Design review of the part built by this model. Coordinates are the model's own, in mm. A direction names the side the tool comes from. Give positions to 0.01 mm unless a question says otherwise; leave off trailing zeros. Order: outer loops, then holes, each group sorted by start corner. A loop starts at its lowest first (then second) coordinate and runs counter-clockwise, first axis right, second up. Notation, with made-up numbers: M 52.5,-28.5 L 95.5,-28.5 A29 cw 95.5,1.5 Z; hole C 24.25,-1.75 d4. An arc over 180 degrees is marked long. Answer as a JSON object with one key per item and string values.
from build123d import *

# Parameters (mm, degrees)
F0_R     = 25
F0_R_2   = 15
F1_DEPTH = 5
F2_DEPTH = 30
F3_R     = 10
F4_DEPTH = 15
F5_R     = 23
F6_DEPTH = 2


with BuildPart() as f1:
    # F0 (on Top) → F1 (new body)
    with BuildSketch(Plane.XY):
        Circle(F0_R)
        Circle(F0_R_2, mode=Mode.SUBTRACT)
    extrude(amount=F1_DEPTH)

    # F0 (on Top) → F2 (join)
    with BuildSketch(Plane.XY):
        Circle(F0_R_2)
    extrude(amount=F2_DEPTH)

    # F3 (on face) → F4 (cut)
    with BuildSketch(Plane.XY.offset(30)):
        Circle(F3_R)
    extrude(amount=-F4_DEPTH, mode=Mode.SUBTRACT)

    # F5 (on face) → F6 (cut)
    with BuildSketch(Plane.XY):
        Circle(F5_R)
    extrude(amount=F6_DEPTH, mode=Mode.SUBTRACT)


solid = f1.part
(1) We need section A-A (y = 0). Write out the cut boundary in (x, z), plus the area to 3 significant figures.
Checked values:
{"outline": "M -25,0 L -23,0 L -23,2 L 23,2 L 23,0 L 25,0 L 25,5 L 15,5 L 15,30 L 10,30 L 10,15 L -10,15 L -10,30 L -15,30 L -15,5 L -25,5 Z", "area": "608 mm^2"}
(2) We need section D-D (z = 9.75). Write out the cut boundary in (x, y).
Checked values:
{"outline": "C 0,0 d30"}
(3) Draft analysis for pull direction X (two halves, no side actions). For faces 4 (the flat face through (11, -11, 5)), 5 (the cylindrical face through (-2.17, -9.76, 22.6)), 6 (the cylindrical face through (-14.985, 0.66, 17.325)), state which applies: +X half, -X half, draft (parallel to the pull), parting line (faces both ways), or undercut.
Checked values:
{"face 4": "draft", "face 5": "undercut", "face 6": "parting line"}
(4) We need section C-C (z = 17.75). Write out the cut boundary in (x, y).
Checked values:
{"outline": "C 0,0 d30; hole C 0,0 d20"}
(5) To check wall thickness, follow L1, parallel to Y at x = 0, z = 0.95; L2, parallel to Z at x = -13, y = -18; L3, parallel to Z at x = 12, y = -1. State the ranges of each line that lie inside material, in increasing order. Write a range as from..to.
Checked values:
{"L1": "y = -25..-23, 23..25", "L2": "z = 2..5", "L3": "z = 2..30"}
(6) Insertion check: pin 1 (1.5 mm diameter, centred on x = -13, y = -17.5, fed in from -Z); pin 2 (10 mm diameter, centred on y = -14.5, z = 13.5, fed in from +X); pin 3 (2 mm diameter, centred on y = -10, z = 22.5, fed in from -X); pin 4 (5 mm diameter, centred on x = -5, y = -14.5, fed in from +Z). Each pin has a flat end and moves straight along its axis. Give the tip position at first contact, or say it passes through.
Checked values:
{"pin 1": "stops at z = 2", "pin 2": "stops at x = 11.61", "pin 3": "stops at x = -12", "pin 4": "stops at z = 30"}
(7) Tool access review of faces 1 (the flat face through (3, -10, 30)), 2 (the flat face through (0, 0, 15)), 3 (the cylindrical face through (-2.994, 22.804, 0.986)): name each direction out of +Z, -Z, +X, -X, +Y, -Y from which nothing blocks a thin tool from reaching the whole face with its end or side.
Checked values:
{"face 1": "+Z, +X, -X, +Y, -Y", "face 2": "+Z", "face 3": "-Z"}
